```python
from build123d import *

# Parameters (mm, degrees)
AUFSATZ_LINEAR_AUSTRAGEN1_DEPTH  = 75
F_3_2_3_2_DURCHMESSER_BOHRUNG3_D = 3.2


with BuildPart() as part:
    # Skizze1 → Aufsatz-Linear austragen1 (new body)
    with BuildSketch(Plane.XY):
        Polygon((-8.5, 0), (8.5, 0), (8.5, 5.5), (5, 5.5), (5, 4), (7, 4), (7, 2), (4, 2), (3.5, 1.5), (-3.5, 1.5), (-4, 2), (-7, 2), (-7, 4), (-5, 4), (-5, 5.5), (-8.5, 5.5), align=None)
    extrude(amount=AUFSATZ_LINEAR_AUSTRAGEN1_DEPTH)

    # Ø3.2 (3.2) Durchmesser Bohrung3 (through all)
    with Locations(Plane(origin=(0, 1.5, 0), x_dir=(1, 0, 0), z_dir=(0, 1, 0))):
        with Locations((0, -80), (0, -20), (0, -140)):
            Hole(F_3_2_3_2_DURCHMESSER_BOHRUNG3_D / 2)


solid = part.part
```
Here's how the part is built. I have some questions about the finished solid (model axes, mm). A direction names the side the tool comes from. Give positions to 0.01 mm unless a question says otherwise; leave off trailing zeros. Order: outer loops, then holes, each group sorted by start corner. A loop starts at its lowest first (then second) coordinate and runs counter-clockwise, first axis right, second up. Notation, with made-up numbers: M 73.25,52.5 L 89.25,52.5 A15 ccw 89.25,69.5 Z; hole C 57,18.25 d11. An arc over 180 degrees is marked long. Use a Markdown table: item, result. Add a question column.
1. Suppose I cut it at D-D (z = 41). List the corners of the cut face in (x, y) for me.
2. Suppose I cut it at A-A (x = 0). List the corners of the cut face in (y, z) for me, and give its area (3 significant figures).
3. If we mould it in two halves opening along X, with no side actions, what happens to faces 4 (the flat face through (-6, 4, 37)), 5 (the flat face through (0, 0, 37)), 6 (the flat face through (6, 2, 37)), 7 (the flat face through (8.5, 3, 37))? For each: +X half, -X half, draft (parallel to the pull), parting line (faces both ways), or undercut.
4. Suppose I cut it at C-C (y = 4.75). List the corners of the cut face in (x, z) for me, and give its area (3 significant figures).
5. Suppose I cut it at B-B (z = 20). List the corners of the cut face in (x, y) for me, and give its area (4 significant figures).
6. On a 3-axis mill with a long thin cutter (end or side, diameter ignored), from which of +Z, -Z, +X, -X, +Y, -Y can I reach the whole of each face in a straight line? I mean faces 1 (the flat face through (7, 3, 37)), 2 (the flat face through (0, 1, 75)), 3 (the flat face through (0, 1.5, 37)). Say none if no direction works.
7. For pin 1 Ø1.5 at (x, z) = (6, 42) entering from -Y; pin 2 Ø2 at (x, z) = (-1.5, 52) entering from +Y, each with a flat end and sliding along its axis, tell me the tip position at first contact or that it passes through.
8. I need wall thicknesses on probe 1 along Z at (x, y) = (0, 0.7); probe 2 along X at (y, z) = (0.4, 20); probe 3 along X at (y, z) = (2.85, 7). Which ranges of each line are inside material? Lowest first, please. Write a range as from..to.
Results list:
| question | item | result |
|---|---|---|
| 1 | outline | M -8.5,0 L 8.5,0 L 8.5,5.5 L 5,5.5 L 5,4 L 7,4 L 7,2 L 4,2 L 3.5,1.5 L -3.5,1.5 L -4,2 L -7,2 L -7,4 L -5,4 L -5,5.5 L -8.5,5.5 Z |
| 2 | outline | M 0,0 L 1.5,0 L 1.5,18.4 L 0,18.4 Z; M 0,21.6 L 1.5,21.6 L 1.5,75 L 0,75 Z |
| 2 | area | 108 mm² |
| 3 | face 4 | undercut |
| 3 | face 5 | draft |
| 3 | face 6 | undercut |
| 3 | face 7 | +X half |
| 4 | outline | M -8.5,0 L -5,0 L -5,75 L -8.5,75 Z; M 5,0 L 8.5,0 L 8.5,75 L 5,75 Z |
| 4 | area | 525 mm² |
| 5 | outline | M -8.5,0 L -1.6,0 L -1.6,1.5 L -3.5,1.5 L -4,2 L -7,2 L -7,4 L -5,4 L -5,5.5 L -8.5,5.5 Z; M 1.6,0 L 8.5,0 L 8.5,5.5 L 5,5.5 L 5,4 L 7,4 L 7,2 L 4,2 L 3.5,1.5 L 1.6,1.5 Z |
| 5 | area | 41.95 mm² |
| 6 | face 1 | +Z, -Z |
| 6 | face 2 | +Z, +X, -X, +Y, -Y |
| 6 | face 3 | +Z, -Z, +Y |
| 7 | pin 1 | stops at y = 0 |
| 7 | pin 2 | stops at y = 1.5 |
| 8 | probe 1 | z = 0..18.4, 21.6..75 |
| 8 | probe 2 | x = -8.5..-1.6, 1.6..8.5 |
| 8 | probe 3 | x = -8.5..-7, 7..8.5 |
